```python
from build123d import *

# Parameters (mm, degrees)
F1_DEPTH  = 25
F2_SIZE   = 1
F3_R      = 10
F4_R      = 5
F5_R      = 2.5
F6_DEPTH  = 25
F5_R_2    = 4.5
F7_DEPTH  = 3
F8_R      = 2.5
F9_DEPTH  = 25
F8_R_2    = 4.5
F10_DEPTH = 3


with BuildPart() as f1:
    # F0 (on Right) → F1 (new body, symmetric)
    with BuildSketch(Plane.YZ):
        Polygon((-115.9307490277, -9.261659597), (-105.9307490277, -9.261659597), (105.9307490277, -9.261659597), (105.9307490277, 9.261659597), (85.9307490277, 9.261659597), (72.102765995, -2.261659597), (68.9018439966, 1.579446801), (78.1204993518, 9.261659597), (53.1204993518, 9.261659597), (39.2925163191, -2.261659597), (36.0915943207, 1.579446801), (45.3102496759, 9.261659597), (20.3102496759, 9.261659597), (6.4822666432, -2.261659597), (3.2813446448, 1.579446801), (12.5, 9.261659597), (-12.5, 9.261659597), (-26.3279830328, -2.261659597), (-29.5289050311, 1.579446801), (-20.3102496759, 9.261659597), (-45.3102496759, 9.261659597), (-59.1382327087, -2.261659597), (-62.339154707, 1.579446801), (-53.1204993518, 9.261659597), (-78.1204993518, 9.261659597), (-91.9484823846, -2.261659597), (-95.1494043829, 1.579446801), (-85.9307490277, 9.261659597), (-105.9307490277, 9.261659597), (-115.9307490277, 9.261659597), align=None)
    extrude(amount=F1_DEPTH, both=True)

    # F2
    f2_edges = [f1.edges().sort_by_distance(p)[0] for p in [
        (0, -85.930749, 9.26166),
        (0, -53.120499, 9.26166),
        (0, -20.31025, 9.26166),
        (0, 12.5, 9.26166),
        (0, 45.31025, 9.26166),
        (0, 78.120499, 9.26166),
    ]]
    chamfer(f2_edges, length=F2_SIZE)

    # F3
    f3_edges = [f1.edges().sort_by_distance(p)[0] for p in [
        (25, -115.930749, 0),
        (-25, -115.930749, 0),
        (25, 105.930749, 0),
        (-25, 105.930749, 0),
    ]]
    fillet(f3_edges, radius=F3_R)

    # F4
    f4_edges = [f1.edges().sort_by_distance(p)[0] for p in [
        (0, 105.930749, 9.26166),
        (22.071068, 103.001817, 9.26166),
        (25, 90.930749, 9.26166),
        (25, 65.120499, 9.26166),
        (25, 32.31025, 9.26166),
        (25, -0.5, 9.26166),
        (25, -33.31025, 9.26166),
        (25, -66.120499, 9.26166),
        (25, -96.430749, 9.26166),
        (22.071068, -113.001817, 9.26166),
        (0, -115.930749, 9.26166),
        (-22.071068, -113.001817, 9.26166),
        (-25, -96.430749, 9.26166),
        (-25, -66.120499, 9.26166),
        (-25, -33.31025, 9.26166),
        (-25, -0.5, 9.26166),
        (-25, 32.31025, 9.26166),
        (-25, 65.120499, 9.26166),
        (-22.071068, 103.001817, 9.26166),
    ]]
    fillet(f4_edges, radius=F4_R)

    # F5 (on face) → F6 (cut)
    with BuildSketch(Plane.XY.offset(9.261659597)):
        with Locations((0, -98.9307490277)):
            Circle(F5_R)
    extrude(amount=-F6_DEPTH, mode=Mode.SUBTRACT)

    # F5 (on face) → F7 (cut)
    with BuildSketch(Plane.XY.offset(9.261659597)):
        with Locations((0, -98.9307490277)):
            Circle(F5_R_2)
        with Locations((0, -98.9307490277)):
            Circle(F5_R, mode=Mode.SUBTRACT)
    extrude(amount=-F7_DEPTH, mode=Mode.SUBTRACT)

    # F8 (on face) → F9 (cut)
    with BuildSketch(Plane.XY.offset(9.261659597)):
        with Locations((0, 93.4307490277)):
            Circle(F8_R)
    extrude(amount=-F9_DEPTH, mode=Mode.SUBTRACT)

    # F8 (on face) → F10 (cut)
    with BuildSketch(Plane.XY.offset(9.261659597)):
        with Locations((0, 93.4307490277)):
            Circle(F8_R_2)
        with Locations((0, 93.4307490277)):
            Circle(F8_R, mode=Mode.SUBTRACT)
    extrude(amount=-F10_DEPTH, mode=Mode.SUBTRACT)


solid = f1.part
```
Input: part model. Units: mm. Frame: model coordinates. A direction names the side the tool comes from. Round coordinates to 2 decimals unless told otherwise and drop trailing zeros. Write each question's results on one line, items separated by ' | '.
Q1. Access query for faces 4 (the face through (0.35, 4.904, -0.368)), 5 (the face through (23.496, -96.449, 7.836)). Directions: +Z, -Z, +X, -X, +Y, -Y. A direction counts if a zero-diameter tool reaches every point of the face in a straight line with its end or side. Return the directions, or none.
Results:
face 4: +X, -X | face 5: +Z, +X, +Y, -Y
Q2. Pin query (flat end, axial travel): P1, Ø8, axis at x = -18, z = 1, coming from the -Y side; P2, Ø6, axis at x = 0, y = 93.43, coming from the +Z side; P3, Ø4, axis at x = 20, z = 5, coming from the +Y side; P4, Ø4, axis at x = 0, y = -98.93, coming from the -Z side. Return the tip coordinate at first contact, or that it passes through.
Results:
P1: stops at y = -115.93 | P2: stops at z = 6.26 | P3: stops at y = 105.45 | P4: passes through
Q3. Line query: line 1 along Y through (x, z) = (0, -3.5); line 2 along Z through (x, y) = (-22.5, -38); line 3 along Z through (x, y) = (-5.5, -23.5) (3 decimals). Output: solid intervals per line, ascending.
Results:
line 1: y = -115.93 to -101.43, -96.43 to 90.93, 95.93 to 105.93 | line 2: z = -9.26 to 8.59 | line 3: z = -9.262 to 0.095, 6.604 to 9.262
Q4. Draft query along Z for faces 1 (the face through (0.21, 104.427, 7.836)), 2 (the face through (0.35, 40.258, 5.051)), 3 (the face through (-0.54, 90.99, -1.39)). Return one class per face: released by +Z, released by -Z, zero draft, split by the parting line, or undercut.
Results:
face 1: released by +Z | face 2: undercut | face 3: zero draft
Q5. Section query A-A (x = 0). State how many separate pieces and enclosed holes the cut face has, and give its area (3 significant figures).
Results:
separate pieces: 3 | enclosed holes: 0 | area: 3,440 mm^2
